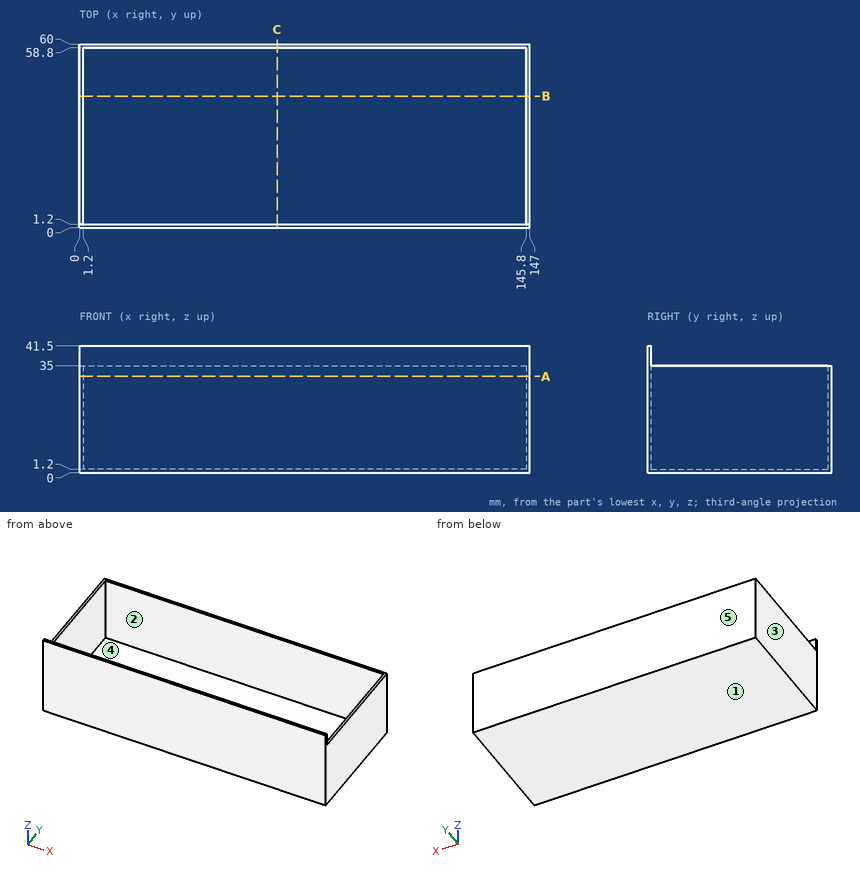
Check sheet for the drawn part. Datum: minimum x, y, z corner. Units: mm. A direction names the side the tool comes from. Coordinates: 2 decimals unless noted, no trailing zeros. Write each loop counter-clockwise with the first axis right and the second up, starting at its lowest first coordinate (ties: lowest second). Pieces come first, ordered by that corner, then holes. Notation, with made-up numbers: (22, 19) - (80, 19) arc R19 ccw to (80, 24) - close; hole circle Ø7 at (-11, 59). An arc over 180 degrees is marked (long way). Answer as a JSON object with one key per item and string values.
(1) Cross-section at A-A on z = 31.5. Record the cut outline in (x, y).
Report:
{"outline": "(0, 0) - (147, 0) - (147, 60) - (0, 60) - close; hole (1.2, 1.2) - (145.8, 1.2) - (145.8, 58.8) - (1.2, 58.8) - close"}
(2) Cross-section at B-B on y = 43. Record the cut outline in (x, z), plus the area to 3 significant figures.
Report:
{"outline": "(0, 0) - (147, 0) - (147, 35) - (145.8, 35) - (145.8, 1.2) - (1.2, 1.2) - (1.2, 35) - (0, 35) - close", "area": "258 mm^2"}
(3) Thickness scan on line 1 along Y through (x, z) = (43.5, 17); line 2 along X through (y, z) = (46, 19); line 3 along Z through (x, y) = (88.5, 48.5). Record the ranges inside material, lowest first.
Report:
{"line 1": "0 to 1.2, 58.8 to 60", "line 2": "0 to 1.2, 145.8 to 147", "line 3": "0 to 1.2"}
(4) Mould release check, pull along X, two halves, no side actions. Record for the marked faces 1, 2 and 3: pulls with the +X half, pulls with the -X half, needs draft (parallel to the pull), parting line crosses it, or undercut.
Report:
{"face 1": "needs draft", "face 2": "undercut", "face 3": "pulls with the -X half"}
(5) Cross-section at C-C on x = 64.5. Record the cut outline in (y, z).
Report:
{"outline": "(0, 0) - (60, 0) - (60, 35) - (58.8, 35) - (58.8, 1.2) - (1.2, 1.2) - (1.2, 41.5) - (0, 41.5) - close"}
(6) Gauge pin test, flat end, axial feed: pin 1 Ø8 at (x, y) = (70.5, 22.5) entering from +Z. Record the tip position at first contact, or that the pin passes through.
Report:
{"pin 1": "z = 1.2"}
(7) Tool access check on the marked faces 4 and 5. Record the directions out of +Z, -Z, +X, -X, +Y, -Y that give a thin tool (end or side, any length) a straight path to the whole face; none if there is none.
Report:
{"face 4": "+Z", "face 5": "+Z, -Z, +X, -X, +Y"}
